Geometry check sheet. Reference: the model listing, model coordinates, mm. Face numbers are marked on the shaded views. A direction names the side the tool comes from. Coordinates: 2 decimals unless noted, no trailing zeros. Loops run counter-clockwise (first coordinate to the right, second up) from the corner with the lowest first, then second, coordinate; pieces in that order, holes last.
from build123d import *

# Parameters (mm, degrees)
F0_W      = 110
F0_H      = 103
F0_R      = 9
F0_W_2    = 80
F0_H_2    = 53
F1_DEPTH  = 21
F2_W      = 100
F2_H      = 93
F2_W_2    = 80
F2_H_2    = 53
F2_R      = 9
F3_DEPTH  = 18
F4_R      = 5
F5_ANGLE  = 180
F7_W      = 51
F7_H      = 16
F3_FACE_W = 93
F3_FACE_H = 18
F8_DEPTH  = 25


with BuildPart() as f1:
    # F0 (on Top) → F1 (new body)
    with BuildSketch(Plane.XY):
        with Locations((-8.2950558215, 3.6971443333)):
            Rectangle(F0_W, F0_H)
        with Locations((28.7049441785, -30.8028556667)):
            Circle(F0_R, mode=Mode.SUBTRACT)
        with Locations((-8.2950558215, 12.6971443333)):
            Rectangle(F0_W_2, F0_H_2, mode=Mode.SUBTRACT)
    extrude(amount=F1_DEPTH)

    # F2 (on face) → F3 (cut)
    with BuildSketch(Plane(origin=(0, 0, 0), x_dir=(1, 0, 0), z_dir=(0, 0, -1))):
        with Locations((-8.2950558215, -3.6971443333)):
            Rectangle(F2_W, F2_H)
        with Locations((-8.2950558215, -12.6971443333)):
            Rectangle(F2_W_2, F2_H_2, mode=Mode.SUBTRACT)
        with Locations((28.7049441785, 30.8028556667)):
            Circle(F2_R, mode=Mode.SUBTRACT)
    extrude(amount=-F3_DEPTH, mode=Mode.SUBTRACT)

    # F4
    f4_edges = [f1.edges().sort_by_distance(p)[0] for p in [
        (-8.295056, -47.802856, 21),
        (46.704944, 3.697144, 21),
        (-8.295056, 55.197144, 21),
        (-63.295056, 3.697144, 21),
    ]]
    fillet(f4_edges, radius=F4_R)


with BuildPart() as f1_1:
    # F5: moved
    add(f1.part.rotate(Axis((46.7049441785, 3.6971443333, 0), (0, 1, 0)), F5_ANGLE))


with BuildPart() as f1_2:
    # F6: moved
    add(f1_1.part.moved(Location((-101.8, -3.3, 22.4))))

    # F7 (on face) + F3_face (on face) → F8 (cut)
    with BuildSketch(Plane.YZ.offset(54.9049441785)):
        with Locations((14.3971443333, 14.4)):
            Rectangle(F7_W, F7_H)
    with BuildSketch(Plane(origin=(49.9049441785, 0.3971443333, 13.4), x_dir=(0, -1, 0), z_dir=(-1, 0, 0))):
        Rectangle(F3_FACE_W, F3_FACE_H)
    extrude(amount=-F8_DEPTH, dir=(1, 0, 0), mode=Mode.SUBTRACT)


solid = f1_2.part
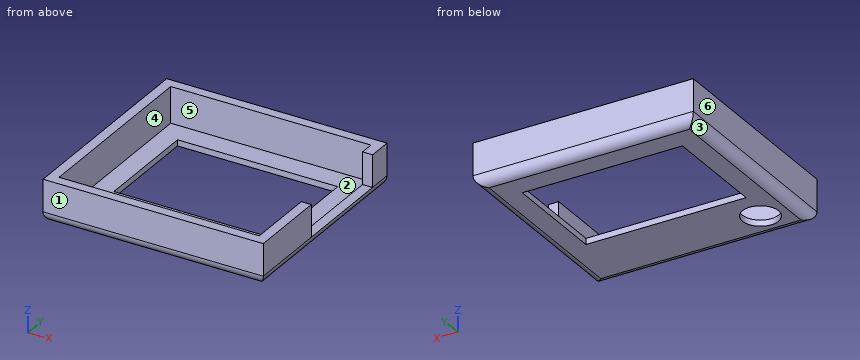
1) Material ranges on probe 1 along X at (y, z) = (-17.5, 7.5); probe 2 along Y at (x, z) = (5, 6.5); probe 3 along Z at (x, y) = (-42, -46), recorded low to high.
Data:
probe 1: x = -55.1 to -50.1, 49.9 to 54.9
probe 2: y = -51.1 to -46.1, 46.9 to 51.9
probe 3: z = 1.4 to 4.4
2) Section check B-B on y = 11.5. Record the cut outline in (x, z), and give its area (3 significant figures).
Data:
outline: (-55.1, 6.4) arc R5 ccw to (-50.1, 1.4) - (-40.1, 1.4) - (-40.1, 4.4) - (-50.1, 4.4) - (-50.1, 22.4) - (-55.1, 22.4) - close; (39.9, 1.4) - (49.9, 1.4) arc R5 ccw to (54.9, 6.4) - (49.9, 6.4) - (49.9, 4.4) - (39.9, 4.4) - close
area: 179 mm2
3) Access from +Z, -Z, +X, -X, +Y, -Y to the whole of each face (thin tool, end or side, straight path). Record for the marked faces 5 and 6.
Data:
face 5: +Z
face 6: +Z, -Z, -X, +Y, -Y
4) Mould release check, pull along Y, two halves, no side actions. Record for the marked faces 1, 2, 3 and 4: +Y half, -Y half, draft (parallel to the pull), parting line (faces both ways), or undercut.
Data:
face 1: -Y half
face 2: undercut
face 3: draft
face 4: undercut
5) Depth check by flat-ended pin: pin 1 (0.9 mm diameter, centred on x = -16, z = 2, fed in from -Y); pin 2 (3.5 mm diameter, centred on y = 15.5, z = 3, fed in from -X); pin 3 (1.5 mm diameter, centred on x = 12.5, z = 2.5, fed in from +Y); pin 4 (5 mm diameter, centred on x = 35.5, y = 0.5, fed in from -Z). Enter the tip coordinate at first touch or a pass-through.
Data:
pin 1: stops at y = -49.17
pin 2: stops at x = -54.81
pin 3: stops at y = 50.78
pin 4: passes through
6) Section check D-D on x = -36.5. Record the cut outline in (y, z).
Data:
outline: (-51.1, 6.4) arc R5 ccw to (-46.1, 1.4) - (-43.08, 1.4) - (-43.08, 4.4) - (-46.1, 4.4) - (-46.1, 22.4) - (-51.1, 22.4) - close; (-25.12, 1.4) - (-17.1, 1.4) - (-17.1, 4.4) - (-25.12, 4.4) - close; (35.9, 1.4) - (46.9, 1.4) arc R5 ccw to (51.9, 6.4) - (51.9, 22.4) - (46.9, 22.4) - (46.9, 4.4) - (35.9, 4.4) - close
7) Section check A-A on x = 0. Record the cut outline in (y, z).
Data:
outline: (-51.1, 6.4) arc R5 ccw to (-46.1, 1.4) - (-17.1, 1.4) - (-17.1, 4.4) - (-46.1, 4.4) - (-46.1, 22.4) - (-51.1, 22.4) - close; (35.9, 1.4) - (46.9, 1.4) arc R5 ccw to (51.9, 6.4) - (51.9, 22.4) - (46.9, 22.4) - (46.9, 4.4) - (35.9, 4.4) - close
8) Section check C-C on z = 14. Record the cut outline in (x, y).
Data:
outline: (-55.1, -51.1) - (54.9, -51.1) - (54.9, -11.1) - (49.9, -11.1) - (49.9, -46.1) - (-50.1, -46.1) - (-50.1, 46.9) - (49.9, 46.9) - (49.9, 39.9) - (54.9, 39.9) - (54.9, 51.9) - (-55.1, 51.9) - close
